Here's the drawing with two shaded views (mm, measured from the low corner). I have some questions. A direction names the side the tool comes from. Coordinates: 2 decimals unless noted, no trailing zeros. Loops run counter-clockwise (first coordinate to the right, second up) from the corner with the lowest first, then second, coordinate; pieces in that order, holes last. Notation, with made-up numbers: (-22.75, 89) - (6.25, 89) arc R33 ccw to (6.25, 128) - close; hole circle Ø3 at (15.25, -1). An arc over 180 degrees is marked (long way). One line per item, written item: value. Start each with the question number.
(1) If we mould it in two halves opening along Z, with no side actions, what happens to the marked faces 1, 2, 3 and 4? For each: pulls with the +Z half, pulls with the -Z half, needs draft (parallel to the pull), parting line crosses it, or undercut.
(2) If we section it at B-B on x = 5: Write out the boundary of the cut face in (y, z).
(3) On a 3-axis mill with a long thin cutter (end or side, diameter ignored), from which of +Z, -Z, +X, -X, +Y, -Y can I reach the whole of each face in a straight line? I mean the marked faces 5, 6, 7 and 8. Say none if no direction works.
(4) If we section it at A-A on z = 7.5: Write out the boundary of the cut face in (x, y), then the cut area to 3 significant figures.
(5) If we section it at D-D on z = 3.5: Write out the boundary of the cut face in (x, y).
(6) If we section it at C-C on y = 2.25: Write out the boundary of the cut face in (x, z).
(7) I'm going to push flat-ended pins straight in: P1, Ø6.5, axis at y = 8.5, z = 10.5, coming from the -X side; P2, Ø3, axis at y = 10.5, z = 10, coming from the +X side; P3, Ø5, axis at x = 5.5, z = 5.5, coming from the +Y side; P4, Ø3, axis at x = 9, y = 2, coming from the -Z side. Where does each tip first touch, or does it pass through?
(8) If I drill on line 1 along X through (y, z) = (4, 8.75); line 2 along Z through (x, y) = (5, 1.4); line 3 along X through (y, z) = (1.75, 4.5), over which ranges is the centre line in solid material (lowest first)? Write a range as from..to.
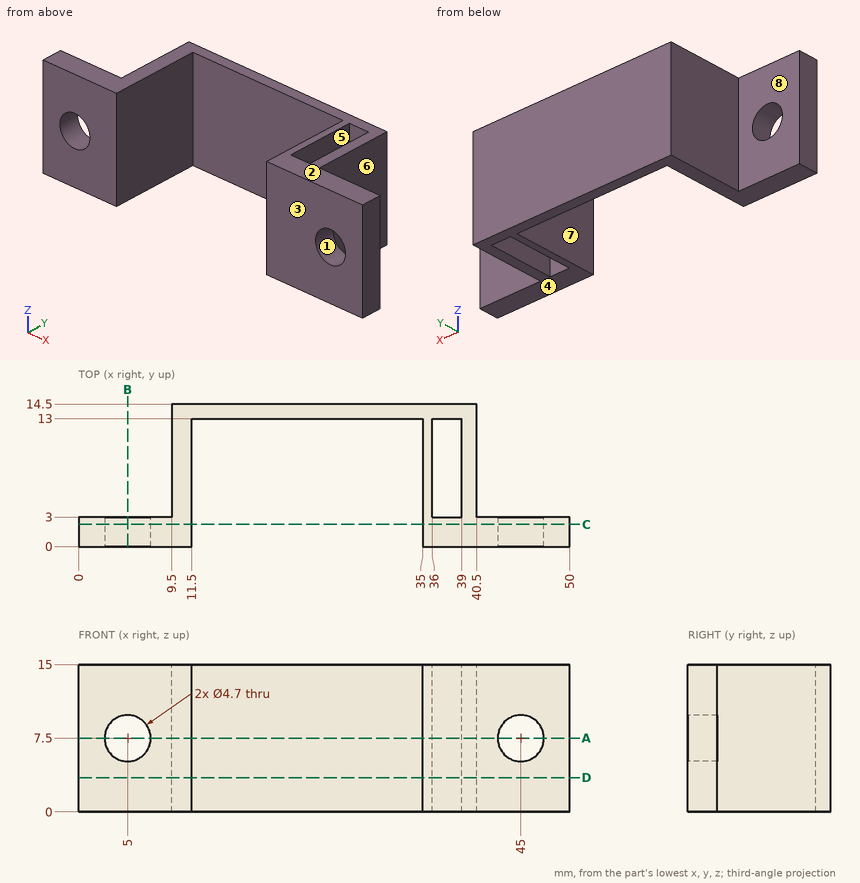
Values:
1. face 1: undercut
1. face 2: pulls with the +Z half
1. face 3: needs draft
1. face 4: pulls with the -Z half
2. outline: (0, 0) - (3, 0) - (3, 5.15) - (0, 5.15) - close; (0, 9.85) - (3, 9.85) - (3, 15) - (0, 15) - close
3. face 5: +Z, -Z
3. face 6: +Z, -Z, +X, +Y
3. face 7: +Z, -Z, -Y
3. face 8: +Z, -Z, -X, +Y
4. outline: (0, 0) - (2.65, 0) - (2.65, 3) - (0, 3) - close; (7.35, 0) - (11.5, 0) - (11.5, 13) - (35, 13) - (35, 0) - (42.65, 0) - (42.65, 3) - (40.5, 3) - (40.5, 14.5) - (9.5, 14.5) - (9.5, 3) - (7.35, 3) - close; (47.35, 0) - (50, 0) - (50, 3) - (47.35, 3) - close; hole (36, 3) - (39, 3) - (39, 13) - (36, 13) - close
4. area: 143 mm2
5. outline: (0, 0) - (11.5, 0) - (11.5, 13) - (35, 13) - (35, 0) - (50, 0) - (50, 3) - (40.5, 3) - (40.5, 14.5) - (9.5, 14.5) - (9.5, 3) - (0, 3) - close; hole (36, 3) - (39, 3) - (39, 13) - (36, 13) - close
6. outline: (0, 0) - (11.5, 0) - (11.5, 15) - (0, 15) - close; (35, 0) - (50, 0) - (50, 15) - (35, 15) - close; hole circle Ø4.7 at (5, 7.5); hole circle Ø4.7 at (45, 7.5)
7. P1: stops at x = 9.5
7. P2: stops at x = 40.5
7. P3: stops at y = 3
7. P4: stops at z = 0
8. line 1: x = 9.5..11.5, 35..36, 39..40.5
8. line 2: z = 0..5.15, 9.85..15
8. line 3: x = 0..11.5, 35..50
